Build history of the part. All positions in model axes, mm. A direction names the side the tool comes from. Give positions to 0.01 mm unless a question says otherwise; leave off trailing zeros. Write each loop counter-clockwise with the first axis right and the second up, starting at its lowest first coordinate (ties: lowest second). Pieces come first, ordered by that corner, then holes. Notation, with made-up numbers: (-15.75, 47.25) -> (12.25, 47.25) arc R10 ccw to (12.25, 56.25) -> close; hole circle Ø4 at (-36, -22). An arc over 180 degrees is marked (long way). Write item = value, one per line. Start each with the question number.
Q1. Mould opens along X. For faces 1 (the face through (1, 13, 0)), 2 (the face through (-5, 9, 7.5)), 3 (the face through (8.7, 11.7, -1.6)), 4 (the face through (-1, 16, 2)) say: pulls with the +X half, pulls with the -X half, needs draft (parallel to the pull), parting line crosses it, or undercut.
Q2. Saw through at B-B, the plane z = 0. List the corners of the cut face in (x, y).
Q3. Drop flat-ended pins along their axis: P1, Ø3.5, axis at y = 18, z = 1, coming from the -X side; P2, Ø5, axis at y = 9.5, z = -3, coming from the -X side; P3, Ø3, axis at y = 12.5, z = -5.5, coming from the +X side; P4, Ø2, axis at x = -10, y = 18.5, coming from the +Z side. Give the stop position or say it passes through.
Q4. Saw through at A-A, the plane y = 0. List the corners of the cut face in (x, z).
Q5. Saw through at D-D, the plane y = 5. List the corners of the cut face in (x, z), then the cut area to 3 significant figures.
Q6. Saw through at C-C, the plane x = -16.5. List the corners of the cut face in (y, z).
Q7. Tool access for faces 5 (the face through (-8.7, 19, 0)), 6 (the face through (4, 18, -2)), 7 (the face through (0, -10, 0)): list every direction of +Z, -Z, +X, -X, +Y, -Y with a clear straight run to the whole face (end or side of a thin tool).
Q8. Wall check: line 1 (Y direction, x = 6.75, z = 0); line 2 (Y direction, x = 1.95, z = 0); line 3 (X direction, y = 15.5, z = 7). Give the ranges that are in metal, low to high.
from build123d import *

# Parameters (mm, degrees)
SKETCH1_R                 = 10
BOSS_EXTRUDE1_DEPTH       = 7.5
FILLET1_R                 = 7
CUT_EXTRUDE1_DEPTH        = 16
CUT_EXTRUDE2_START        = 3
SKETCH3_R                 = 4.60375
CUT_EXTRUDE2_DEPTH        = 15
F_8_CLEARANCE_HOLE1_D     = 4.9149
F_8_CLEARANCE_HOLE1_DEPTH = 3
F_8_32_TAPPED_HOLE1_D     = 3.4544
F_8_CLEARANCE_HOLE2_D     = 4.3053
F_8_CLEARANCE_HOLE2_DEPTH = 15


with BuildPart() as part:
    # Sketch1 → Boss-Extrude1 (new body, symmetric)
    with BuildSketch(Plane.XY):
        with BuildLine():
            Line((-8.7, 20.749939759), (-8.7, 9.290956753))
            Line((-8.7, 9.290956753), (-18.627272727, 3.96543954))
            ThreePointArc((-18.627272727, 3.96543954), (-21, 0), (-18.627272727, -3.96543954))
            Line((-18.627272727, -3.96543954), (-5.814545455, -10.838868075))
            ThreePointArc((-5.814545455, -10.838868075), (9.872829559, -7.336023207), (8.7, 8.694826048))
            Line((8.7, 8.694826048), (8.7, 20.749939759))
            ThreePointArc((8.7, 20.749939759), (0, 22.5), (-8.7, 20.749939759))
        make_face()
        Circle(SKETCH1_R, mode=Mode.SUBTRACT)
    extrude(amount=BOSS_EXTRUDE1_DEPTH, both=True)

    # Fillet1
    fillet1_edges = [part.edges().sort_by_distance(p)[0] for p in [
        (8.7, 8.694826048, 0),
        (-8.7, 9.290956753, 0),
    ]]
    fillet(fillet1_edges, radius=FILLET1_R)

    # Sketch2 → Cut-Extrude1 (cut, through all)
    with BuildSketch(Plane.XY.offset(7.5)):
        with BuildLine():
            Line((-1, 22.477766793), (-1, 9.949874371))
            ThreePointArc((-1, 9.949874371), (0, 10), (1, 9.949874371))
            Line((1, 9.949874371), (1, 22.477766793))
            ThreePointArc((1, 22.477766793), (0, 22.5), (-1, 22.477766793))
        make_face()
    extrude(amount=-CUT_EXTRUDE1_DEPTH, mode=Mode.SUBTRACT)

    # Sketch3 → Cut-Extrude2 (cut)
    with BuildSketch(Plane(origin=(1, 0, 0), x_dir=(0, 0, -1), z_dir=(1, 0, 0)).offset(CUT_EXTRUDE2_START)):
        with Locations(Location((0, 16.213820582, 0), (0, 0, 80.166973696))):  # turned: the seam where the file's is
            Circle(SKETCH3_R)
    extrude(amount=CUT_EXTRUDE2_DEPTH, mode=Mode.SUBTRACT)

    # #8 Clearance Hole1
    with Locations(Plane(origin=(4, 0, 0), x_dir=(0, 0, -1), z_dir=(1, 0, 0))):
        with Locations((0, 16.213820582)):
            Hole(F_8_CLEARANCE_HOLE1_D / 2, depth=F_8_CLEARANCE_HOLE1_DEPTH)

    # #8-32 Tapped Hole1 (through all)
    with Locations(Plane(origin=(-1, 1.097851263, -6.242435486), x_dir=(0, 0, 1), z_dir=(1, 0, 0))):
        with Locations((6.242435486, -15.115969319)):
            Hole(F_8_32_TAPPED_HOLE1_D / 2)

    # #8 Clearance Hole2
    with Locations(Plane.XY.offset(7.5)):
        with Locations((-16.5, 0)):
            Hole(F_8_CLEARANCE_HOLE2_D / 2, depth=F_8_CLEARANCE_HOLE2_DEPTH)


solid = part.part
Report:
q1.face_1 = undercut
q1.face_2 = needs draft
q1.face_3 = pulls with the +X half
q1.face_4 = undercut
q2.outline = (-18.63, -3.97) -> (-5.81, -10.84) arc R12.3 ccw to (10.01, 7.15) arc R7 cw to (8.7, 11.22) -> (8.7, 11.61) -> (4, 11.61) -> (4, 13.76) -> (1, 13.76) -> (1, 9.95) arc R10 cw (long way) to (-1, 9.95) -> (-1, 14.49) -> (-8.7, 14.49) -> (-8.7, 13.48) arc R7 cw to (-12.39, 7.31) -> (-18.63, 3.97) arc R4.5 ccw to start; (-8.7, 17.94) -> (-1, 17.94) -> (-1, 22.48) arc R22.5 ccw to (-8.7, 20.75) -> close; (1, 18.67) -> (4, 18.67) -> (4, 20.82) -> (8.54, 20.82) arc R22.5 ccw to (1, 22.48) -> close; hole circle Ø4.31 at (-16.5, 0)
q3.P1 = -8.7
q3.P2 = -12.97
q3.P3 = 8.7
q3.P4 = through
q4.outline = (-21, -7.5) -> (-18.65, -7.5) -> (-18.65, 7.5) -> (-21, 7.5) -> close; (-14.35, -7.5) -> (-10, -7.5) -> (-10, 7.5) -> (-14.35, 7.5) -> close; (10, -7.5) -> (12.3, -7.5) -> (12.3, 7.5) -> (10, 7.5) -> close
q5.outline = (-16.7, -7.5) -> (-8.66, -7.5) -> (-8.66, 7.5) -> (-16.7, 7.5) -> close; (8.66, -7.5) -> (11.24, -7.5) -> (11.24, 7.5) -> (8.66, 7.5) -> close
q5.area = 159 mm2
q6.outline = (-5.11, -7.5) -> (-2.15, -7.5) -> (-2.15, 7.5) -> (-5.11, 7.5) -> close; (2.15, -7.5) -> (5.11, -7.5) -> (5.11, 7.5) -> (2.15, 7.5) -> close
q7.face_5 = +Z, -Z, -X, +Y
q7.face_6 = +X
q7.face_7 = +Z, -Z
q8.line_1 = -10.28 to -7.38, 7.38 to 11.61, 20.82 to 21.46
q8.line_2 = -12.14 to -9.81, 9.81 to 13.76, 18.67 to 22.42
q8.line_3 = -8.7 to -1, 1 to 8.7
